Build history of the part. All positions in model axes, mm. Face numbers are marked on the shaded views. Round coordinates to 2 decimals unless told otherwise and drop trailing zeros. Loops run counter-clockwise (first coordinate to the right, second up) from the corner with the lowest first, then second, coordinate; pieces in that order, holes last.
from build123d import *

# Parameters (mm, degrees)
F0_W      = 620
F0_H      = 415
F1_DEPTH  = 5
F2_W      = 620
F2_H      = 5
F3_DEPTH  = 175
F5_D      = 5
F7_D      = 5
F9_D      = 5
F11_D     = 5
F15_D     = 5
F17_D     = 5
F19_D     = 5
F19_DEPTH = 11
F20_D     = 5
F20_DEPTH = 11


with BuildPart() as f1:
    # F0 (on Top) → F1 (new body)
    with BuildSketch(Plane.XY):
        Rectangle(F0_W, F0_H)
    extrude(amount=F1_DEPTH)

    # F2 (on face) → F3 (join)
    with BuildSketch(Plane.XY.offset(5)):
        with Locations((0, -205)):
            Rectangle(F2_W, F2_H)
    extrude(amount=F3_DEPTH)

    # F5 (through all)
    with Locations(Plane.XZ.offset(207.5)):
        with Locations((300, 170)):
            Hole(F5_D / 2)

    # F7 (through all)
    with Locations(Plane.XZ.offset(207.5)):
        with Locations((300, 150)):
            Hole(F7_D / 2)

    # F9 (through all)
    with Locations(Plane.XZ.offset(207.5)):
        with Locations((-250, 170)):
            Hole(F9_D / 2)

    # F11 (through all)
    with Locations(Plane.XZ.offset(207.5)):
        with Locations((-250, 150)):
            Hole(F11_D / 2)

    # F15 (through all)
    with Locations(Plane(origin=(0, 0, 0), x_dir=(1, 0, 0), z_dir=(0, 0, -1))):
        with Locations((290, 195)):
            Hole(F15_D / 2)

    # F17 (through all)
    with Locations(Plane(origin=(0, 0, 0), x_dir=(1, 0, 0), z_dir=(0, 0, -1))):
        with Locations((-290, 195)):
            Hole(F17_D / 2)

    # F19
    with Locations(Plane.XZ.offset(207.5)):
        with Locations((285, 25)):
            Hole(F19_D / 2, depth=F19_DEPTH)

    # F20
    with Locations(Plane.XZ.offset(207.5)):
        with Locations((-300, 20), (-280, 20), (-300, 160), (-280, 160)):
            Hole(F20_D / 2, depth=F20_DEPTH)


solid = f1.part
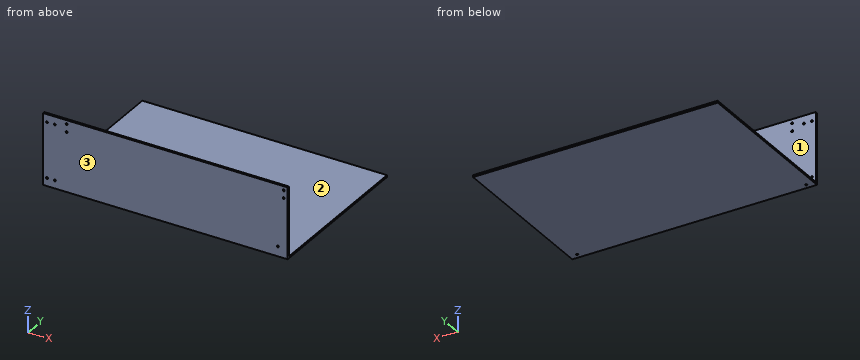
(1) Pin check, flat tips, straight feed: P1, Ø8, axis at x = 300, z = 170, coming from the +Y side; P2, Ø8, axis at x = -231.5, y = -100, coming from the +Z side; P3, Ø4.5, axis at x = -300, z = 160, coming from the +Y side. Stop position of each tip, or through.
Responses:
P1: stops at y = -202.5
P2: stops at z = 5
P3: passes through
(2) Pull direction Y, two halves, no side cores. Call the marked faces 1, 2 and 3: +Y half, -Y half, draft (parallel to the pull), parting line (faces both ways), or undercut.
Responses:
face 1: +Y half
face 2: draft
face 3: -Y half
(3) Slice it at B-B on z = 67. List the corners of the cut face in (x, y), plus the area to 3 significant figures.
Responses:
outline: (-310, -207.5) - (310, -207.5) - (310, -202.5) - (-310, -202.5) - close
area: 3,100 mm2
(4) Slice it at C-C on y = 50. List the corners of the cut face in (x, z).
Responses:
outline: (-310, 0) - (310, 0) - (310, 5) - (-310, 5) - close
(5) Probe line 1 (Z direction, x = -250, y = -206); line 2 (Z direction, x = 285, y = -205); line 3 (Z direction, x = -280, y = -203). List the from-to ranges inside material, lowest first.
Responses:
line 1: z = 0 to 147.5, 152.5 to 167.5, 172.5 to 180
line 2: z = 0 to 22.5, 27.5 to 180
line 3: z = 0 to 17.5, 22.5 to 157.5, 162.5 to 180
(6) Slice it at A-A on x = -213. List the corners of the cut face in (y, z).
Responses:
outline: (-207.5, 0) - (207.5, 0) - (207.5, 5) - (-202.5, 5) - (-202.5, 180) - (-207.5, 180) - close
